Verification items for the finished model (mm, model axes). Face numbers are marked on the shaded views. A direction names the side the tool comes from. Round coordinates to 2 decimals unless told otherwise and drop trailing zeros. Order: outer loops, then holes, each group sorted by start corner. A loop starts at its lowest first (then second) coordinate and runs counter-clockwise, first axis right, second up. Notation, with made-up numbers: (-26, 28.25) -> (-7, 28.25) arc R25 ccw to (-7, 42.25) -> close; hole circle Ø3 at (-23, 46). An arc over 180 degrees is marked (long way). Return JSON: item names as keys, results as strings. Group by question number.
Item 1: Sectioned sample at A-A on y = -47.5. Record the cut outline in (x, z), plus the area to 3 significant figures.
Item 2: Access from +Z, -Z, +X, -X, +Y, -Y to the whole of each face (thin tool, end or side, straight path). Record for the marked faces 4, 5, 6, 7 and 8.
Item 3: Sectioned sample at D-D on x = -27.5. Record the cut outline in (y, z), plus the area to 3 significant figures.
Item 4: Depth check by flat-ended pin: pin 1 Ø12 at (x, y) = (-54, -33.5) entering from -Z; pin 2 Ø12 at (y, z) = (-42.5, -4.5) entering from +X; pin 3 Ø10 at (x, y) = (-32.5, 24.5) entering from +Z; pin 4 Ø6 at (x, z) = (-9.5, 10) entering from -Y. Enter the tip coordinate at first touch or a pass-through.
Item 5: Scan lines: probe 1 along X at (y, z) = (-28.5, 16); probe 2 along X at (y, z) = (-3, -9.5); probe 3 along X at (y, z) = (13, 16.5). Record each from-to range of solid material in increasing order. Write a range as from..to.
Item 6: Sectioned sample at B-B on x = -96.5. Record the cut outline in (y, z).
Item 7: Draft check along X on the marked faces 1, 2 and 3. Enter one of: pulls with the +X half, pulls with the -X half, needs draft (parallel to the pull), parting line crosses it, or undercut.
Item 8: Sectioned sample at C-C on z = -1.5. Record the cut outline in (x, y), plus the area to 3 significant figures.
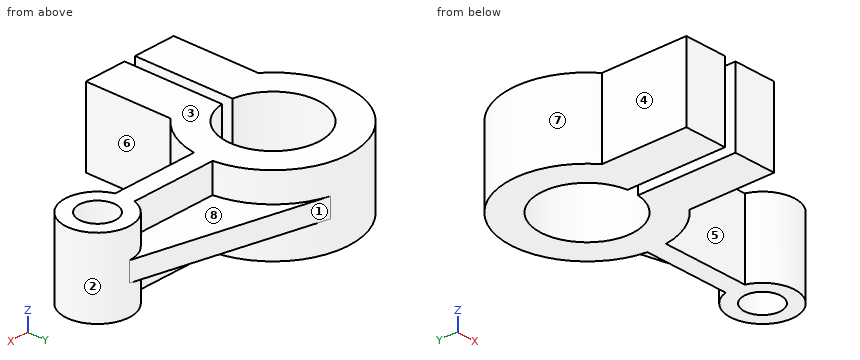
```python
from build123d import *

# Parameters (mm, degrees)
BOSS_EXTRUDE1_DEPTH = 20
SKETCH2_3_R         = 9.427573189
CUT_EXTRUDE1_DEPTH  = 20
RIB14_REACH         = 148.086
SKETCH4_WALL_W      = 387.490512318
SKETCH4_WALL_H      = 10


with BuildPart() as part:
    # Sketch2 → Boss-Extrude1 (new, symmetric)
    with BuildSketch(Plane.XY):
        with BuildLine():
            Line((-47.815474815, 9.850065555), (-3.248646384, 9.850065555))
            ThreePointArc((-3.248646384, 9.850065555), (29.513615172, 5.671147892), (-3.023551525, 0))
            Line((-3.023551525, 0), (-47.906799475, 0))
            ThreePointArc((-47.906799475, 0), (-52.615248836, -14.092543666), (-62.182699169, -25.460620745))
            Line((-62.182699169, -25.460620745), (-62.182699169, -69.710398251))
            Line((-62.182699169, -69.710398251), (-84.182699169, -69.710398251))
            Line((-84.182699169, -69.710398251), (-84.182699169, -18.657805359))
            ThreePointArc((-84.182699169, -18.657805359), (-87.182699169, 29.424189114), (-90.182699169, -18.657805359))
            Line((-90.182699169, -18.657805359), (-90.182699169, -69.710398251))
            Line((-90.182699169, -69.710398251), (-112.182699169, -69.710398251))
            Line((-112.182699169, -69.710398251), (-112.182699169, -25.460620745))
            ThreePointArc((-112.182699169, -25.460620745), (-106.243534032, 40.035259864), (-47.815474815, 9.850065555))
        make_face()
    extrude(amount=BOSS_EXTRUDE1_DEPTH, both=True)

    # Sketch2<3> → Cut-Extrude1 (cut, symmetric)
    with BuildSketch(Plane.XY):
        with Locations((12.817300831, 5.289601749)):
            Circle(SKETCH2_3_R)
    extrude(amount=CUT_EXTRUDE1_DEPTH, both=True, mode=Mode.SUBTRACT)

    # Sketch4 wall → Rib14 (add, up to next)
    with BuildSketch(Plane(origin=(-32.547275207, 32.905370949, 0), x_dir=(0.972252919165, -0.233932172167, 0), z_dir=(0.233932172167, 0.972252919165, 0)), mode=Mode.PRIVATE) as rib14_sk1:
        Rectangle(SKETCH4_WALL_W, SKETCH4_WALL_H)
    rib14_tool1 = extrude(rib14_sk1.sketch, amount=-RIB14_REACH, mode=Mode.PRIVATE) - part.part
    add(rib14_tool1.solids().sort_by_distance((-32.547275207, 32.905370949, 0))[0])


solid = part.part
```
Recorded:
{
 "1": {"outline": "(-112.18, -20) -> (-90.18, -20) -> (-90.18, 20) -> (-112.18, 20) -> close; (-84.18, -20) -> (-62.18, -20) -> (-62.18, 20) -> (-84.18, 20) -> close", "area": "1,760 mm²"},
 "2": {"face 4": "+Z, -Z, -X, -Y", "face 5": "+Z, -Z, -Y", "face 6": "+Z, -Z, +X, -Y", "face 7": "none", "face 8": "+Z, +Y"},
 "3": {"outline": "(0, -20) -> (9.85, -20) -> (9.85, -5) -> (31.69, -5) -> (31.69, 5) -> (9.85, 5) -> (9.85, 20) -> (0, 20) -> close", "area": "612 mm²"},
 "4": {"pin 1": "through", "pin 2": "x = -62.18", "pin 3": "z = 5", "pin 4": "y = 0"},
 "5": {"probe 1": "-112.18..-90.18, -84.18..-62.18", "probe 2": "-125.94..-109.85, -64.52..-48.43, -1.68..8.33, 17.31..27.32", "probe 3": "-126.06..-110.05, -64.31..-48.31, -2..7.39, 18.24..27.63"},
 "6": {"outline": "(-69.71, -20) -> (-16.97, -20) -> (-16.97, 20) -> (-69.71, 20) -> close; (27.55, -20) -> (43.81, -20) -> (43.81, 20) -> (27.55, 20) -> close"},
 "7": {"face 1": "pulls with the +X half", "face 2": "undercut", "face 3": "needs draft"},
 "8": {"outline": "(-112.18, -69.71) -> (-90.18, -69.71) -> (-90.18, -18.66) arc R24.13 cw (long way) to (-84.18, -18.66) -> (-84.18, -69.71) -> (-62.18, -69.71) -> (-62.18, -25.46) arc R39.63 ccw to (-47.91, 0) -> (-3.02, 0) arc R16.7 ccw (long way) to (12.82, 21.99) -> (-77.91, 43.82) arc R39.63 ccw to (-112.18, -25.46) -> close; hole circle Ø18.86 at (12.82, 5.29)", "area": "6,950 mm²"}
}
